For this review, take the finished solid that the model builds, in its own axes (mm). A direction names the side the tool comes from. Coordinates: 2 decimals unless noted, no trailing zeros. Write each loop counter-clockwise with the first axis right and the second up, starting at its lowest first coordinate (ties: lowest second). Pieces come first, ordered by that corner, then holes. Notation, with made-up numbers: (-3.75, 76) - (40.25, 76) arc R19 ccw to (40.25, 110) - close; hole circle Ø5 at (70.25, -27). An arc over 180 degrees is marked (long way). Write each question's results on one line, items separated by ' | '.
from build123d import *

# Parameters (mm, degrees)
F0_W      = 23.368
F0_H      = 13.97
F1_DEPTH  = 2.794
F2_W      = 23.368
F2_H      = 2.794
F3_DEPTH  = 14.986
F3_FACE_W = 23.368
F3_FACE_H = 2.794
F4_DEPTH  = 2.794
F5_W      = 23.368
F5_H      = 2.794
F6_DEPTH  = 13.97
F8_DEPTH  = 25.4
F9_W      = 23.368
F9_H      = 3.81
F10_DEPTH = 25.4


with BuildPart() as f1:
    # F0 (on Top) → F1 (new body)
    with BuildSketch(Plane.XY):
        Rectangle(F0_W, F0_H)
    extrude(amount=F1_DEPTH)

    # F2 (on face) → F3 (join)
    with BuildSketch(Plane(origin=(0, 0, 0), x_dir=(1, 0, 0), z_dir=(0, 0, -1))):
        with Locations((0, 8.382)):
            Rectangle(F2_W, F2_H)
    extrude(amount=-F3_DEPTH)

    # F3_face (on face) → F4 (join)
    with BuildSketch(Plane(origin=(0, -8.382, 14.986), x_dir=(1, 0, 0), z_dir=(0, 0, 1))):
        Rectangle(F3_FACE_W, F3_FACE_H)
    extrude(amount=F4_DEPTH)

    # F5 (on face) → F6 (join)
    with BuildSketch(Plane(origin=(0, -6.985, 0), x_dir=(-1, 0, 0), z_dir=(0, 1, 0))):
        with Locations((0, 16.383)):
            Rectangle(F5_W, F5_H)
    extrude(amount=F6_DEPTH)

    # F7 (on face) → F8 (cut)
    with BuildSketch(Plane.XZ.offset(9.779)):
        Polygon((-8.636, 10.795), (-11.684, 10.795), (-11.684, 8.89), (-11.684, 6.985), (-8.636, 6.985), align=None)
    extrude(amount=-F8_DEPTH, mode=Mode.SUBTRACT)

    # F9 (on face) → F10 (join)
    with BuildSketch(Plane.XZ.offset(9.779)):
        with Locations((0, 15.875)):
            Rectangle(F9_W, F9_H)
    extrude(amount=F10_DEPTH)


solid = f1.part
Q1. Take a section at A-A on y = -0.5. State the section outline as (x, z) points, plus the area to 3 significant figures.
Results found:
outline: (-11.68, 0) - (11.68, 0) - (11.68, 2.79) - (-11.68, 2.79) - close; (-11.68, 14.99) - (11.68, 14.99) - (11.68, 17.78) - (-11.68, 17.78) - close | area: 131 mm2
Q2. Mouldability with a two-part tool opening along Z and no side actions: class faces 1 (the face through (0, 6.985, 1)), 2 (the face through (0, -6.985, 9)), 3 (the face through (0, 0, 2.794)), 4 (the face through (0, -2, 0)) as pulls with the +Z half, pulls with the -Z half, needs draft (parallel to the pull), parting line crosses it, or undercut.
Results found:
face 1: needs draft | face 2: undercut | face 3: undercut | face 4: pulls with the -Z half
Q3. Take a section at C-C on x = 4.75. State the section outline as (y, z) points (3 decimals).
Results found:
outline: (-35.179, 13.97) - (-9.779, 13.97) - (-9.779, 0) - (6.985, 0) - (6.985, 2.794) - (-6.985, 2.794) - (-6.985, 14.986) - (6.985, 14.986) - (6.985, 17.78) - (-35.179, 17.78) - close
Q4. Wall thickness on line 1 along Z through (x, y) = (9.5, -3); line 2 along Z through (x, y) = (2.25, -13.5); line 3 along Y through (x, z) = (5.75, 11.75) (3 decimals): over which ranges is each line inside the solid? List them lowest first. Write a range as from..to.
Results found:
line 1: 0..2.79, 14.99..17.78 | line 2: 13.97..17.78 | line 3: -9.779..-6.985
Q5. Take a section at B-B on y = -7.5. State the section outline as (x, z) points (3 decimals).
Results found:
outline: (-11.684, 0) - (11.684, 0) - (11.684, 17.78) - (-11.684, 17.78) - (-11.684, 10.795) - (-8.636, 10.795) - (-8.636, 6.985) - (-11.684, 6.985) - close
Q6. For pin 1 (7 mm diameter, centred on x = 3, z = 9.5, fed in from -Y); pin 2 (3 mm diameter, centred on x = 1.5, y = -11.5, fed in from -Z); pin 3 (11 mm diameter, centred on x = 4, y = -1, fed in from -Z); pin 4 (2 mm diameter, centred on y = -9, z = 8.5, fed in from -X), all flat-tipped, find the tip position at first contact; note any pin that passes through.
Results found:
pin 1: y = -9.78 | pin 2: z = 13.97 | pin 3: z = 0 | pin 4: x = -8.64
Q7. Take a section at D-D on z = 9.25. State the section outline as (x, y) points (3 decimals).
Results found:
outline: (-8.636, -9.779) - (11.684, -9.779) - (11.684, -6.985) - (-8.636, -6.985) - close
Q8. For faces 5 (the face through (-10, -8, 6.985)), 6 (the face through (0, 6.985, 16)), 7 (the face through (0, 0, 14.986)), 8 (the face through (0, -22, 13.97)), 9 (the face through (0, -35.179, 16)), list the 3-axis set-ups (+Z, -Z, +X, -X, +Y, -Y) from which the entire face can be reached by the end or side of a thin tool; tool diameter is ignored.
Results found:
face 5: -X, +Y, -Y | face 6: +Z, -Z, +X, -X, +Y | face 7: +X, -X, +Y | face 8: -Z, +X, -X, -Y | face 9: +Z, -Z, +X, -X, -Y
